Input: dimensioned drawing with shaded views. Units: mm. Origin: part minimum x, y, z. A direction names the side the tool comes from. Coordinates: 2 decimals unless noted, no trailing zeros. Loops run counter-clockwise (first coordinate to the right, second up) from the corner with the lowest first, then second, coordinate; pieces in that order, holes last. Notation, with made-up numbers: M 59.5,62.25 L 79.5,62.25 A21 cw 79.5,83.25 Z; hole C 75,3.25 d11. An arc over 180 degrees is marked long. Write item = value, one per line. Start each with the question number.
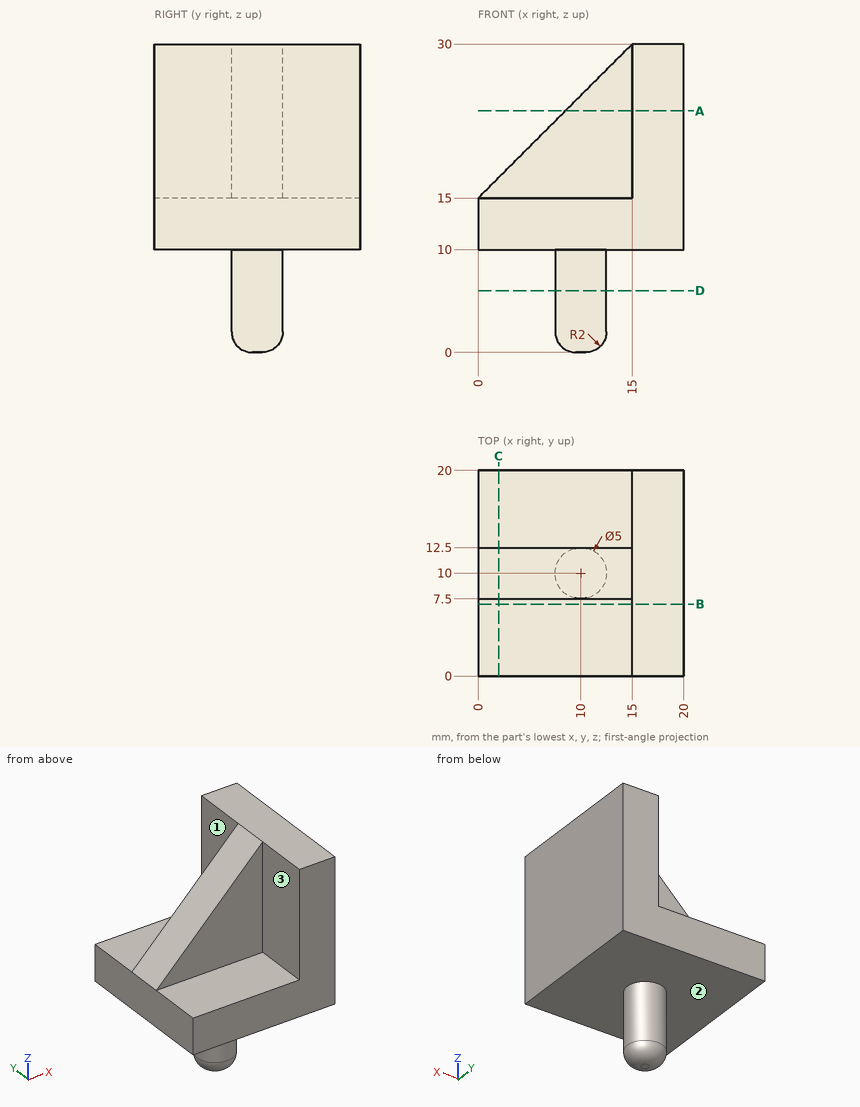
Item 1: Reachability of the marked faces 1, 2 and 3 from +Z, -Z, +X, -X, +Y, -Y: full face, straight path, thin tool, end or side. Return the list, or none.
Item 2: First-contact query: pin 1 (1.5 mm diameter, centred on x = 12, y = 4.5, fed in from +Z); pin 2 (2 mm diameter, centred on y = 5.5, z = 19.5, fed in from -X); pin 3 (1.5 mm diameter, centred on x = 11, y = 5, fed in from -Z); pin 4 (4.5 mm diameter, centred on x = 7, z = 25.5, fed in from -Y). Flat tips, straight axial feed; report the tip coordinate or a pass-through.
Item 3: Section query C-C (x = 2). Return the cut outline in (y, z), plus the area to 3 significant figures.
Item 4: Section query A-A (z = 23.5). Return the cut outline in (x, y).
Item 5: Section query B-B (y = 7). Return the cut outline in (x, z), plus the area to 3 significant figures.
Item 6: Line query: line 1 (Z direction, x = 7.5, y = 2.25); line 2 (Z direction, x = 15.5, y = 17.5); line 3 (Y direction, x = 12.75, z = 18). Output: solid intervals per line, ascending. Write a range as from..to.
Item 7: Section query D-D (z = 6). Return the cut outline in (x, y).
Verdict:
q1.face_1 = +Z, -X, +Y
q1.face_2 = -Z
q1.face_3 = +Z, -X, -Y
q2.pin_1 = 15
q2.pin_2 = 15
q2.pin_3 = 10
q2.pin_4 = through
q3.outline = M 0,10 L 20,10 L 20,15 L 12.5,15 L 12.5,17 L 7.5,17 L 7.5,15 L 0,15 Z
q3.area = 110 mm2
q4.outline = M 8.5,7.5 L 15,7.5 L 15,0 L 20,0 L 20,20 L 15,20 L 15,12.5 L 8.5,12.5 Z
q5.outline = M 0,10 L 20,10 L 20,30 L 15,30 L 15,15 L 0,15 Z
q5.area = 175 mm2
q6.line_1 = 10..15
q6.line_2 = 10..30
q6.line_3 = 7.5..12.5
q7.outline = C 10,10 d5
